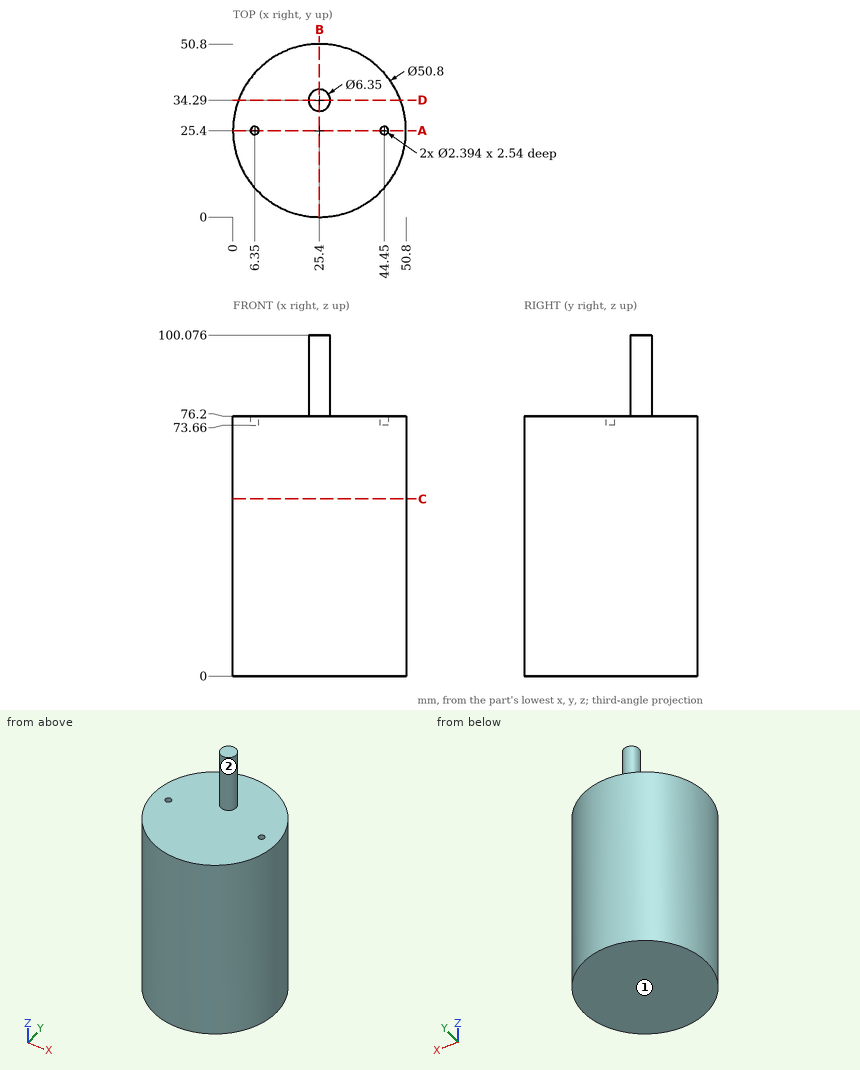
Could you check a few things on this drawing? It's one solid part, dimensions in mm from its lowest x, y, z. A direction names the side the tool comes from. Give positions to 0.01 mm unless a question says otherwise; leave off trailing zeros. Write each loop counter-clockwise with the first axis right and the second up, starting at its lowest first coordinate (ties: lowest second). Pieces come first, ordered by that corner, then holes. Notation, with made-up numbers: (52, -22) - (90, -22) arc R23 ccw to (90, -11) - close; hole circle Ø6 at (74.25, 84). An arc over 180 degrees is marked (long way). Use CSV: the item, a comma, the result in double quotes. Start each with the question number.
Item 1: I want a section at B-B, the plane x = 25.4. Please give me the cut outline in (y, z) (1 decimal).
Item 2: I want a section at C-C, the plane z = 52. Please give me the cut outline in (x, y).
Item 3: I'm going to push flat-ended pins straight in: pin 1 (4 mm diameter, centred on x = 44.45, y = 25.4, fed in from +Z); pin 2 (2 mm diameter, centred on x = 38, z = 16.5, fed in from -Y); pin 3 (6 mm diameter, centred on x = 9, z = 52, fed in from +Y). Where does each tip first touch, or does it pass through?
Item 4: I want a section at A-A, the plane y = 25.4. Please give me the cut outline in (x, z), then the cut area to 3 significant figures.
Item 5: If I drill on line 1 along Z through (x, y) = (39, 36); line 2 along Y through (x, z) = (44.45, 74.6) (1 decimal); line 3 along Y through (x, z) = (6, 75) (1 decimal), over which ranges is the centre line in solid material (lowest first)?
Item 6: For the marked faces 1 and 2, which set-ups out of +Z, -Z, +X, -X, +Y, -Y let a thin tool reach every point of the face, with its end or its side?
Item 7: I want a section at D-D, the plane y = 34.29. Please give me the cut outline in (x, z) (1 decimal), then the cut area to 3 significant figures.
Findings:
1,outline,"(0, 0) - (50.8, 0) - (50.8, 76.2) - (37.5, 76.2) - (37.5, 100.1) - (31.1, 100.1) - (31.1, 76.2) - (0, 76.2) - close"
2,outline,"circle Ø50.8 at (25.4, 25.4)"
3,pin 1,"stops at z = 76.2"
3,pin 2,"stops at y = 2.8"
3,pin 3,"stops at y = 46.98"
4,outline,"(0, 0) - (50.8, 0) - (50.8, 76.2) - (45.65, 76.2) - (45.65, 73.66) - (43.25, 73.66) - (43.25, 76.2) - (7.55, 76.2) - (7.55, 73.66) - (5.15, 73.66) - (5.15, 76.2) - (0, 76.2) - close"
4,area,"3,860 mm2"
5,line 1,"z = 0 to 76.2"
5,line 2,"y = 8.6 to 24.2, 26.6 to 42.2"
5,line 3,"y = 9 to 24.3, 26.5 to 41.8"
6,face 1,"-Z, +X, -X, +Y, -Y"
6,face 2,"+Z"
7,outline,"(1.6, 0) - (49.2, 0) - (49.2, 76.2) - (28.6, 76.2) - (28.6, 100.1) - (22.2, 100.1) - (22.2, 76.2) - (1.6, 76.2) - close"
7,area,"3,780 mm2"
